Model file for the job. Use its own axes, mm. Give positions to 0.01 mm unless a question says otherwise; leave off trailing zeros. Loops run counter-clockwise (first coordinate to the right, second up) from the corner with the lowest first, then second, coordinate; pieces in that order, holes last. Notation, with made-up numbers: M 68,72 L 106,72 A31 cw 106,96 Z; hole C -8.75,67.25 d6. An arc over 180 degrees is marked long. Answer in a Markdown table with one row per item.
```python
from build123d import *

# Parameters (mm, degrees)
SKETCH_1_W          = 586.5
SKETCH_1_H          = 640
EXTRUDE_1_DEPTH     = 3
CUT_EXTRUDE_1_DEPTH = 3
SKETCH_3_R          = 140
CUT_EXTRUDE_2_DEPTH = 3
SKETCH_4_R          = 4.5
CUT_EXTRUDE_3_DEPTH = 869.09633682
SKETCH_5_R          = 3.25
CUT_EXTRUDE_4_DEPTH = 869.09633682


with BuildPart() as part:
    # 스케치1 → 보스-돌출1 (new body)
    with BuildSketch(Plane(origin=(0, 0, 0), x_dir=(1, 0, 0), z_dir=(0, 1, 0))):
        with Locations((293.25, 320)):
            Rectangle(SKETCH_1_W, SKETCH_1_H)
    extrude(amount=EXTRUDE_1_DEPTH)

    # 스케치2 → 컷-돌출1 (cut)
    with BuildSketch(Plane(origin=(0, 3, 0), x_dir=(1, 0, 0), z_dir=(0, 1, 0))):
        with BuildLine():
            Line((0, 470.5), (105, 470.5))
            ThreePointArc((105, 470.5), (112.071067812, 467.571067812), (115, 460.5))
            Line((115, 460.5), (115, 179.5))
            ThreePointArc((115, 179.5), (112.071067812, 172.428932188), (105, 169.5))
            Line((105, 169.5), (0, 169.5))
            Line((0, 169.5), (0, 470.5))
        make_face()
    extrude(amount=-CUT_EXTRUDE_1_DEPTH, mode=Mode.SUBTRACT)

    # 스케치3 → 컷-돌출2 (cut)
    with BuildSketch(Plane(origin=(0, 3, 0), x_dir=(1, 0, 0), z_dir=(0, 1, 0))):
        with Locations(Location((365.5, 320, 0), (0, 0, 270))):
            Circle(SKETCH_3_R)
    extrude(amount=-CUT_EXTRUDE_2_DEPTH, mode=Mode.SUBTRACT)

    # 스케치4 → 컷-돌출3 (cut, through all)
    with BuildSketch(Plane(origin=(0, 3, 0), x_dir=(1, 0, 0), z_dir=(0, 1, 0))):
        with Locations(Location((259.433982822, 426.066017178, 0), (0, 0, 270))):
            Circle(SKETCH_4_R)
        with Locations(Location((471.566017178, 426.066017178, 0), (0, 0, 270))):
            Circle(SKETCH_4_R)
        with Locations(Location((471.566017178, 213.933982822, 0), (0, 0, 270))):
            Circle(SKETCH_4_R)
        with Locations(Location((259.433982822, 213.933982822, 0), (0, 0, 270))):
            Circle(SKETCH_4_R)
    extrude(amount=-CUT_EXTRUDE_3_DEPTH, mode=Mode.SUBTRACT)

    # 스케치5 → 컷-돌출4 (cut, through all)
    with BuildSketch(Plane(origin=(0, 3, 0), x_dir=(1, 0, 0), z_dir=(0, 1, 0))):
        with Locations(Location((59, 631.5, 0), (0, 0, 270))):
            Circle(SKETCH_5_R)
        with Locations(Location((505.5, 631.5, 0), (0, 0, 270))):
            Circle(SKETCH_5_R)
        with Locations(Location((185.5, 490, 0), (0, 0, 270))):
            Circle(SKETCH_5_R)
        with Locations(Location((577, 490, 0), (0, 0, 270))):
            Circle(SKETCH_5_R)
        with Locations(Location((577, 150, 0), (0, 0, 90))):
            Circle(SKETCH_5_R)
        with Locations(Location((185.5, 150, 0), (0, 0, 90))):
            Circle(SKETCH_5_R)
        with Locations(Location((505.5, 8.5, 0), (0, 0, 90))):
            Circle(SKETCH_5_R)
        with Locations(Location((59, 8.5, 0), (0, 0, 90))):
            Circle(SKETCH_5_R)
    extrude(amount=-CUT_EXTRUDE_4_DEPTH, mode=Mode.SUBTRACT)


solid = part.part
```
(1) Saw through at A-A, the plane x = 365.5. Give the cut face in (y, z).
Established:
| item | result |
|---|---|
| outline | M 0,-640 L 3,-640 L 3,-460 L 0,-460 Z; M 0,-180 L 3,-180 L 3,0 L 0,0 Z |
(2) Mould opens along X. For faces 1 (the flat face through (224, 3, -324)), 2 (the cylindrical face through (483.55, 1.52, -244.74)) say: pulls with the +X half, pulls with the -X half, needs draft (parallel to the pull), parting line crosses it, or undercut.
Established:
| item | result |
|---|---|
| face 1 | needs draft |
| face 2 | undercut |
(3) Flat gauge pin, fed straight in: P1, Ø0.9, axis at y = 1.5, z = -264, coming from the -X side. Where does the tip first touch, or does it go through?
Established:
| item | result |
|---|---|
| P1 | stops at x = 115 |
(4) Saw through at B-B, the plane z = -267. Give the cut face in (x, y).
Established:
| item | result |
|---|---|
| outline | M 115,0 L 235.92,0 L 235.92,3 L 115,3 Z; M 495.08,0 L 586.5,0 L 586.5,3 L 495.08,3 Z |
(5) Wall check: L1, parallel to Z at x = 185.5, y = 0.7; L2, parallel to X at y = 2.2, z = -8.5; L3, parallel to X at y = 2.65, z = -324. Give the ranges that are in metal, low to high.
Established:
| item | result |
|---|---|
| L1 | z = -640 to -493.25, -486.75 to -153.25, -146.75 to 0 |
| L2 | x = 0 to 55.75, 62.25 to 502.25, 508.75 to 586.5 |
| L3 | x = 115 to 225.56, 505.44 to 586.5 |
(6) Saw through at C-C, the plane y = 0.5. Count the separate pieces of the cut face and the enclosed holes in it, and give its area (3 significant figures).
Established:
| item | result |
|---|---|
| separate pieces | 1 |
| enclosed holes | 13 |
| area | 279,000 mm2 |
